Build history of the part. All positions in model axes, mm. Round coordinates to 2 decimals unless told otherwise and drop trailing zeros. Order: outer loops, then holes, each group sorted by start corner. A loop starts at its lowest first (then second) coordinate and runs counter-clockwise, first axis right, second up. Notation, with made-up numbers: (17.25, 76) -> (31.25, 76) arc R24 cw to (31.25, 95) -> close; hole circle Ø5 at (18.5, 24). An arc over 180 degrees is marked (long way). Write item = value, one per line.
from build123d import *

# Parameters (mm, degrees)
F0_W     = 2.5
F0_H     = 12
F1_DEPTH = 2
F2_R     = 0.5


with BuildPart() as f1:
    # F0 (on Top) → F1 (new body)
    with BuildSketch(Plane.XY):
        Polygon((-1, -13), (-1, -25), (1, -25), (1, -1), (1, 1), (1, 13), (1, 25), (-1, 25), (-1, 1), (-1, -1), align=None)
        with Locations((-2.25, -7)):
            Rectangle(F0_W, F0_H)
        Polygon((1, 1), (1, -1), (4, -1), (4, -25), (6, -25), (6, 1), (3.5, 1), align=None)
        Polygon((-3.5, -1), (-1, -1), (-1, 1), (-4, 1), (-4, 25), (-6, 25), (-6, -1), align=None)
        with Locations((2.25, 7)):
            Rectangle(F0_W, F0_H)
    extrude(amount=F1_DEPTH)

    # F2
    f2_edges = [f1.edges().sort_by_distance(p)[0] for p in [
        (-1, -25, 1),
        (-1, 1, 1),
        (-6, -1, 1),
        (1, -25, 1),
        (4, -25, 1),
        (6, -25, 1),
        (1, -1, 1),
        (4, -1, 1),
        (6, 1, 1),
        (-4, 1, 1),
        (-6, 25, 1),
        (-4, 25, 1),
        (-1, 25, 1),
        (1, 25, 1),
        (3.5, 13, 1),
        (-3.5, -13, 1),
        (-3.5, -1, 1),
        (3.5, 1, 1),
        (-1, -13, 1),
        (1, 13, 1),
    ]]
    fillet(f2_edges, radius=F2_R)


solid = f1.part
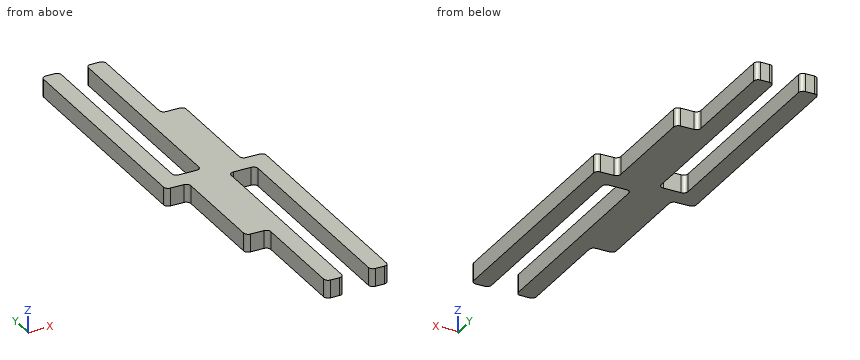
Q1. Cut at C-C, the plane x = -2.5. List the corners of the cut face in (y, z).
Check values:
outline = (-13, 0) -> (1, 0) -> (1, 2) -> (-13, 2) -> close
Q2. Cut at D-D, the plane x = -5. List the corners of the cut face in (y, z), and give its area (3 significant figures).
Check values:
outline = (-1, 0) -> (25, 0) -> (25, 2) -> (-1, 2) -> close
area = 52.0 mm²
Q3. Cut at B-B, the plane y = -18.5. List the corners of the cut face in (x, z).
Check values:
outline = (-1, 0) -> (1, 0) -> (1, 2) -> (-1, 2) -> close; (4, 0) -> (6, 0) -> (6, 2) -> (4, 2) -> close
Q4. Flat gauge pins, fed straight in: pin 1 (1.2 mm diameter, centred on x = 4.5, z = 1.5, fed in from +Y); pin 2 (0.6 mm diameter, centred on y = -4.5, z = 1.5, fed in from -X). Where does each tip first touch, or does it go through?
Check values:
pin_1 = 1.01
pin_2 = -3.5
Q5. Cut at A-A, the plane y = 2.5. List the corners of the cut face in (x, z), and give its area (3 significant figures).
Check values:
outline = (-6, 0) -> (-4, 0) -> (-4, 2) -> (-6, 2) -> close; (-1, 0) -> (3.5, 0) -> (3.5, 2) -> (-1, 2) -> close
area = 13.0 mm²
Q6. Probe probe 1 along X at (y, z) = (14, 0.8); probe 2 along X at (y, z) = (-16, 1.4); probe 3 along Y at (x, z) = (3, 0.75). List the from-to ranges inside material, lowest first.
Check values:
probe_1 = -6 to -4, -1 to 1
probe_2 = -1 to 1, 4 to 6
probe_3 = -1 to 13
